Design review of the part shown in the three views and the two pictorial views. Dimensions are in mm from the part's minimum x, y and z. A direction names the side the tool comes from. Give positions to 0.01 mm unless a question says otherwise; leave off trailing zeros. Order: outer loops, then holes, each group sorted by start corner. A loop starts at its lowest first (then second) coordinate and runs counter-clockwise, first axis right, second up. Notation, with made-up numbers: (-39.5, -38.5) - (-4.5, -38.5) arc R24 ccw to (-4.5, -4.5) - close; hole circle Ø10 at (28.5, 49.25). An arc over 180 degrees is marked (long way). Put each result on its own line as item: value.
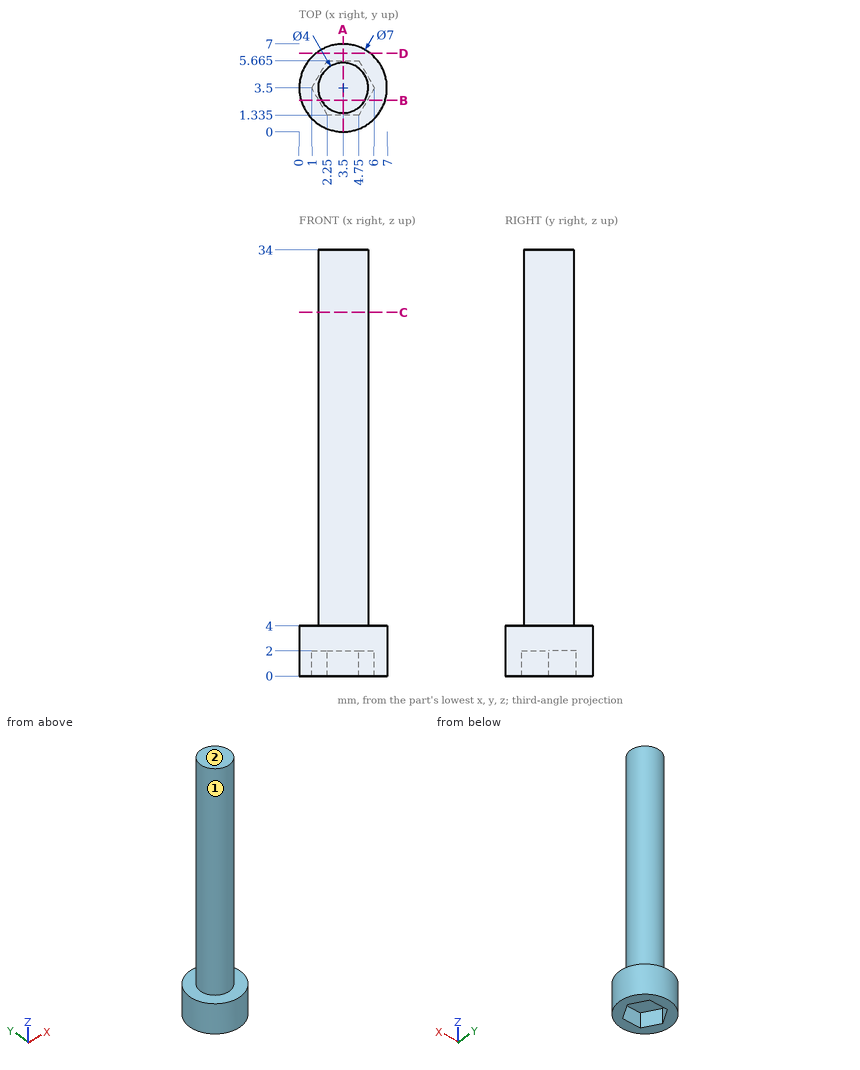
(1) Take a section at C-C, the plane z = 29. Write out the cut boundary in (x, y), then the cut area to 3 significant figures.
The answers:
outline: circle Ø4 at (3.5, 3.5)
area: 12.6 mm^2
(2) Take a section at D-D, the plane y = 6.25. Write out the cut boundary in (x, z) (3 decimals).
The answers:
outline: (1.335, 0) - (5.665, 0) - (5.665, 4) - (1.335, 4) - close
(3) Wall thickness on L1, parallel to Z at x = 5.5, y = 1.25; L2, parallel to Y at x = 6.25, z = 2.5 (1 decimal); L3, parallel to Z at x = 2.5, y = 3: over which ranges is each line inside the solid? List them lowest first.
The answers:
L1: 0 to 4
L2: 1.3 to 5.7
L3: 2 to 34
(4) Take a section at B-B, the plane y = 2.5. Write out the cut boundary in (x, z).
The answers:
outline: (0.15, 0) - (1.58, 0) - (1.58, 2) - (5.42, 2) - (5.42, 0) - (6.85, 0) - (6.85, 4) - (5.23, 4) - (5.23, 34) - (1.77, 34) - (1.77, 4) - (0.15, 4) - close
(5) Take a section at A-A, the plane x = 3.5. Write out the cut boundary in (y, z) (3 decimals), then the cut area to 3 significant figures.
The answers:
outline: (0, 0) - (1.335, 0) - (1.335, 2) - (5.665, 2) - (5.665, 0) - (7, 0) - (7, 4) - (5.5, 4) - (5.5, 34) - (1.5, 34) - (1.5, 4) - (0, 4) - close
area: 139 mm^2
(6) For the marked faces 1 and 2, list the 3-axis set-ups (+Z, -Z, +X, -X, +Y, -Y) from which the entire face can be reached by the end or side of a thin tool; tool diameter is ignored.
The answers:
face 1: +Z
face 2: +Z, +X, -X, +Y, -Y
(7) Clearance check with flat-ended pins moving along their axes: pin 1 Ø1.5 at (y, z) = (5, 26) entering from +X; pin 2 Ø3 at (x, z) = (6, 7) entering from -Y; pin 3 Ø0.6 at (x, z) = (4, 1) entering from -Y. State where each tip first meets the part, or that it passes through.
The answers:
pin 1: x = 5.35
pin 2: y = 1.77
pin 3: y = 0.01
